Check sheet for the modelled part. Datum: model origin and axes. Units: mm. A direction names the side the tool comes from. Round coordinates to 2 decimals unless told otherwise and drop trailing zeros. Loops run counter-clockwise (first coordinate to the right, second up) from the corner with the lowest first, then second, coordinate; pieces in that order, holes last. Notation, with made-up numbers: (-12.75, 71) - (23.25, 71) arc R32 cw to (23.25, 100) - close; hole circle Ø3 at (5, 23). An arc over 180 degrees is marked (long way). Return JSON: item names as keys, results as strings.
from build123d import *

# Parameters (mm, degrees)
SKETCH_W        = 30
SKETCH_H        = 10
PAD_DEPTH       = 13
SKETCH001_W     = 20
SKETCH001_H     = 1.5
POCKET_DEPTH    = 10
SKETCH002_W     = 1.5
SKETCH002_H     = 3.5
POCKET001_DEPTH = 10
POCKET002_DEPTH = 10.001
CHAMFER_SIZE    = 1
SKETCH004_R     = 3
POCKET003_DEPTH = 3
CHAMFER001_SIZE = 0.4


with BuildPart() as part:
    # Sketch → Pad (new body)
    with BuildSketch(Plane.XZ):
        with Locations((0, 5)):
            Rectangle(SKETCH_W, SKETCH_H)
    extrude(amount=PAD_DEPTH)

    # Sketch001 (on Face6 of Pad) → Pocket (cut)
    with BuildSketch(Plane.XZ.offset(13)):
        with Locations((0, 5.75)):
            Rectangle(SKETCH001_W, SKETCH001_H)
    extrude(amount=-POCKET_DEPTH, mode=Mode.SUBTRACT)

    # Sketch002 (on Face5 of Pocket) → Pocket001 (cut)
    with BuildSketch(Plane.XZ.offset(13)):
        with Locations((-6.75, 8.25)):
            Rectangle(SKETCH002_W, SKETCH002_H)
        with Locations((-2.25, 8.25)):
            Rectangle(SKETCH002_W, SKETCH002_H)
        with Locations((2.25, 8.25)):
            Rectangle(SKETCH002_W, SKETCH002_H)
        with Locations((6.75, 8.25)):
            Rectangle(SKETCH002_W, SKETCH002_H)
    extrude(amount=-POCKET001_DEPTH, mode=Mode.SUBTRACT)

    # Sketch003 (on Face6 of Pocket001) → Pocket002 (cut, through all)
    with BuildSketch(Plane(origin=(0, 0, 10), x_dir=(-1, 0, 0), z_dir=(0, 0, 1))):
        Polygon((-15, 7.25), (-12.25, 4.25), (-12.25, 0), (-15, 0), align=None)
        Polygon((15, 7.25), (12.25, 4.25), (12.25, 0), (15, 0), align=None)
    extrude(amount=-POCKET002_DEPTH, mode=Mode.SUBTRACT)

    # Chamfer
    chamfer_edges = [part.edges().sort_by_distance(p)[0] for p in [
        (-7.5, -13, 8.25),
        (-8.75, -13, 6.5),
        (-10, -13, 5.75),
        (0, -13, 5),
        (10, -13, 5.75),
        (8.75, -13, 6.5),
        (7.5, -13, 8.25),
        (6, -13, 8.25),
        (4.5, -13, 6.5),
        (3, -13, 8.25),
        (1.5, -13, 8.25),
        (0, -13, 6.5),
        (-1.5, -13, 8.25),
        (-3, -13, 8.25),
        (-4.5, -13, 6.5),
        (-6, -13, 8.25),
    ]]
    chamfer(chamfer_edges, length=CHAMFER_SIZE)

    # Sketch004 (on Face6 of Chamfer) → Pocket003 (cut)
    with BuildSketch(Plane(origin=(0, 0, 0), x_dir=(1, 0, 0), z_dir=(0, 0, -1))):
        with Locations((-7, 8)):
            Circle(SKETCH004_R)
        with Locations((7, 8)):
            Circle(SKETCH004_R)
    extrude(amount=-POCKET003_DEPTH, mode=Mode.SUBTRACT)

    # Chamfer001
    chamfer001_edges = [part.edges().sort_by_distance(p)[0] for p in [
        (-13.625, -5.75, 0),
        (-15, -10.125, 0),
        (-12.25, -2.125, 0),
        (0, -13, 0),
        (0, 0, 0),
        (15, -10.125, 0),
        (12.25, -2.125, 0),
        (13.625, -5.75, 0),
        (-10, -8, 0),
        (4, -8, 0),
        (-15, -13, 5),
        (-12.25, 0, 5),
        (12.25, 0, 5),
        (15, -13, 5),
        (-11.75, -13, 10),
        (-8, -12.5, 10),
        (-7.5, -7.5, 10),
        (-6.75, -3, 10),
        (-6, -7.5, 10),
        (-5.5, -12.5, 10),
        (-4.5, -13, 10),
        (-3.5, -12.5, 10),
        (-3, -7.5, 10),
        (-2.25, -3, 10),
        (-1.5, -7.5, 10),
        (-1, -12.5, 10),
        (0, -13, 10),
        (1, -12.5, 10),
        (1.5, -7.5, 10),
        (2.25, -3, 10),
        (3, -7.5, 10),
        (3.5, -12.5, 10),
        (4.5, -13, 10),
        (5.5, -12.5, 10),
        (6, -7.5, 10),
        (6.75, -3, 10),
        (7.5, -7.5, 10),
        (8, -12.5, 10),
        (11.75, -13, 10),
        (15, -10.125, 10),
        (13.625, -5.75, 10),
        (12.25, -2.125, 10),
        (0, 0, 10),
        (-12.25, -2.125, 10),
        (-13.625, -5.75, 10),
        (-15, -10.125, 10),
    ]]
    chamfer(chamfer001_edges, length=CHAMFER001_SIZE)


solid = part.part
Q1. Sectioned sample at B-B (y = -8). State how many separate pieces and enclosed holes the cut face has, plus the area to 3 significant figures.
Answer key:
{"separate pieces": "4", "enclosed holes": "0", "area": "212 mm²"}
Q2. Tool access check on faces 5 (the face through (-4.14, -8.9, 1.68)), 6 (the face through (-13.4, -5.8, 9.8)), 7 (the face through (8, -12.5, 8.4)), 8 (the face through (10, -8, 6)), 9 (the face through (-12.25, -2, 5)). Record the directions out of +Z, -Z, +X, -X, +Y, -Y that give a thin tool (end or side, any length) a straight path to the whole face; none if there is none.
Answer key:
{"face 5": "-Z", "face 6": "+Z, -X, +Y", "face 7": "+Z, -Y", "face 8": "-Y", "face 9": "+Z, -Z, -X, +Y"}
Q3. Scan lines: probe 1 along X at (y, z) = (-11.5, 8.75); probe 2 along X at (y, z) = (-8, 2); probe 3 along Z at (x, y) = (-9, -3.5). Record each from-to range of solid material in increasing order. Write a range as [from, to].
Answer key:
{"probe 1": "x = [-15, -7.5], [-6, -3], [-1.5, 1.5], [3, 6], [7.5, 15]", "probe 2": "x = [-15, -10], [-4, 4], [10, 15]", "probe 3": "z = [0, 5], [6.5, 10]"}
Q4. Sectioned sample at C-C (z = 5.5). Enter the section's corners in (x, y), plus the area to 3 significant figures.
Answer key:
{"outline": "(-15, -12.6) - (-14.6, -13) - (-11, -13) - (-10, -12) - (-10, -3) - (10, -3) - (10, -12) - (11, -13) - (14.6, -13) - (15, -12.6) - (15, -7.25) - (12.25, -4.25) - (12.25, -0.4) - (11.85, 0) - (-11.85, 0) - (-12.25, -0.4) - (-12.25, -4.25) - (-15, -7.25) - close", "area": "157 mm²"}
Q5. Sectioned sample at A-A (x = 7). Enter the section's corners in (y, z).
Answer key:
{"outline": "(-13, 0.4) - (-12.6, 0) - (-11.4, 0) - (-11, 0.4) - (-11, 3) - (-5, 3) - (-5, 0.4) - (-4.6, 0) - (-0.4, 0) - (0, 0.4) - (0, 9.6) - (-0.4, 10) - (-2.6, 10) - (-3, 9.6) - (-3, 5) - (-12, 5) - (-13, 4) - close"}
Q6. Draft check along Z on faces 1 (the face through (-6, -8, 8)), 2 (the face through (0, -12.4, 6.9)), 3 (the face through (8.15, -12.37, 9.8)), 4 (the face through (7, -8, 3)). Enter one of: released by +Z, released by -Z, zero draft, split by the parting line, or undercut.
Answer key:
{"face 1": "zero draft", "face 2": "undercut", "face 3": "released by +Z", "face 4": "released by -Z"}
Q7. Depth check by flat-ended pin: P1, Ø5, axis at x = 7, y = -8, coming from the +Z side; P2, Ø0.8, axis at x = -8.5, y = -6.5, coming from the -Z side; P3, Ø1.5, axis at y = -3, z = 5, coming from the +X side; P4, Ø1.2, axis at y = -6.5, z = 6, coming from the -X side. Enter the tip coordinate at first touch or a pass-through.
Answer key:
{"P1": "stops at z = 10", "P2": "stops at z = 3", "P3": "stops at x = 12.25", "P4": "stops at x = -14.86"}
